Part model, mm, in its own coordinate system. Face numbers are marked on the shaded views. A direction names the side the tool comes from. Coordinates: 2 decimals unless noted, no trailing zeros. Write each loop counter-clockwise with the first axis right and the second up, starting at its lowest first coordinate (ties: lowest second). Pieces come first, ordered by that corner, then holes. Notation, with made-up numbers: (36, -13.5) - (42, -13.5) arc R18 ccw to (42, 10.5) - close; hole circle Ø6 at (5.25, 28.5). An arc over 180 degrees is marked (long way). Use one line per item in the form item = value. Start each with the question number.
from build123d import *

# Parameters (mm, degrees)
BOSS_EXTRUDE1_DEPTH = 15
CHAMFER1_SIZE       = 3
CHAMFER2_SIZE       = 3
SKETCH2_R           = 2.5
CUT_EXTRUDE1_DEPTH  = 37
SKETCH3_R           = 1.5
CUT_EXTRUDE2_DEPTH  = 6


with BuildPart() as part:
    # Sketch1 → Boss-Extrude1 (new body)
    with BuildSketch(Plane.XY):
        Polygon((8.117882489, 6.249295775), (12.117882489, 6.249295775), (12.117882489, -17.750704225), (-12.882117511, -17.750704225), (-12.882117511, 6.249295775), (-8.882117511, 6.249295775), (-8.882117511, -13.750704225), (8.117882489, -13.750704225), align=None)
    extrude(amount=BOSS_EXTRUDE1_DEPTH)

    # Chamfer1
    chamfer1_edges = [part.edges().sort_by_distance(p)[0] for p in [
        (-8.882117511, -13.750704225, 7.5),
    ]]
    chamfer(chamfer1_edges, length=CHAMFER1_SIZE)

    # Chamfer2
    chamfer2_edges = [part.edges().sort_by_distance(p)[0] for p in [
        (8.117882489, -13.750704225, 7.5),
    ]]
    chamfer(chamfer2_edges, length=CHAMFER2_SIZE)

    # Sketch2 → Cut-Extrude1 (cut)
    with BuildSketch(Plane.ZY.offset(12.882117511)):
        with Locations(Location((7.5, 1.249295775, 0), (0, 0, 90))):
            Circle(SKETCH2_R)
    extrude(amount=-CUT_EXTRUDE1_DEPTH, mode=Mode.SUBTRACT)

    # Sketch3 → Cut-Extrude2 (cut)
    with BuildSketch(Plane.XZ.offset(17.750704225)):
        with Locations(Location((-9.882117511, 12, 0), (0, 0, 270))):
            Circle(SKETCH3_R)
        with Locations(Location((-9.882117511, 3, 0), (0, 0, 90))):
            Circle(SKETCH3_R)
        with Locations(Location((9.117882489, 12, 0), (0, 0, 90))):
            Circle(SKETCH3_R)
        with Locations(Location((9.117882489, 3, 0), (0, 0, 270))):
            Circle(SKETCH3_R)
    extrude(amount=-CUT_EXTRUDE2_DEPTH, mode=Mode.SUBTRACT)


solid = part.part
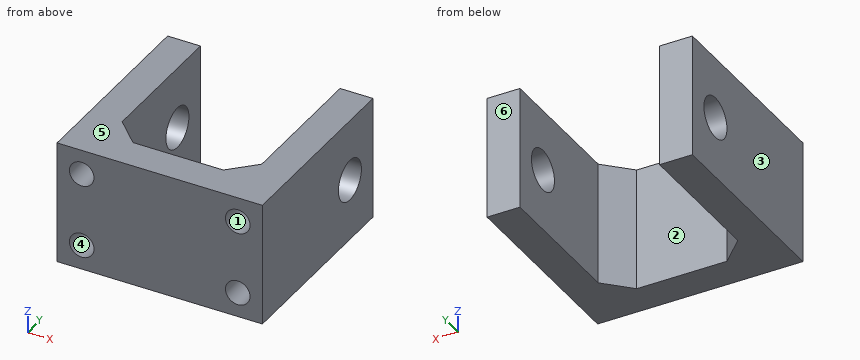
Q1. Pin check, flat tips, straight feed: P1, Ø2.5, axis at x = -10.5, z = 12, coming from the -Y side; P2, Ø0.9, axis at x = 9.5, z = 11.5, coming from the -Y side; P3, Ø9, axis at x = 2, z = 6.5, coming from the +Y side. Stop position of each tip, or through.
Q2. Slice it at B-B (y = 2). List the corners of the cut face in (x, z), plus the area to 3 significant figures.
Q3. Which spindle directions (+Z, -Z, +X, -X, +Y, -Y) get a long thin tool onto all of the face, cutting with end or side? Do the marked faces 1, 2 and 3. Say none if no direction does.
Q4. Slice it at D-D (x = 8.5). List the corners of the cut face in (y, z), plus the area to 3 significant figures.
Q5. Slice it at C-C (z = 3). List the corners of the cut face in (x, y), plus the area to 3 significant figures.
Q6. Slice it at A-A (z = 7.5). List the corners of the cut face in (x, y), plus the area to 3 significant figures.
Q7. Drill centre lines: probe 1 along X at (y, z) = (-14.2, 12); probe 2 along X at (y, z) = (-8, 8); probe 3 along X at (y, z) = (-13.2, 3). Where is each one in solid material? Low to high.
Q8. Mould opens along Z. For the marked faces 4, 5 and 6 say: released by +Z, released by -Z, zero draft, split by the parting line, or undercut.
Solution:
q1.P1 = -17.75
q1.P2 = -11.75
q1.P3 = -12.37
q2.outline = (-12.88, 0) - (-8.88, 0) - (-8.88, 5.12) - (-12.88, 5.12) - close; (-12.88, 9.88) - (-8.88, 9.88) - (-8.88, 15) - (-12.88, 15) - close; (8.12, 0) - (12.12, 0) - (12.12, 5.12) - (8.12, 5.12) - close; (8.12, 9.88) - (12.12, 9.88) - (12.12, 15) - (8.12, 15) - close
q2.area = 81.8 mm2
q3.face_1 = -Y
q3.face_2 = +Z, -Z, +Y
q3.face_3 = +Z, -Z, -X, +Y, -Y
q4.outline = (-17.75, 0) - (6.25, 0) - (6.25, 15) - (-17.75, 15) - (-17.75, 13.37) - (-11.75, 13.37) - (-11.75, 10.63) - (-17.75, 10.63) - (-17.75, 4.37) - (-11.75, 4.37) - (-11.75, 1.63) - (-17.75, 1.63) - close; hole circle Ø5 at (1.25, 7.5)
q4.area = 308 mm2
q5.outline = (-12.88, -17.75) - (-11.38, -17.75) - (-11.38, -11.75) - (-8.38, -11.75) - (-8.38, -17.75) - (7.62, -17.75) - (7.62, -11.75) - (10.62, -11.75) - (10.62, -17.75) - (12.12, -17.75) - (12.12, 6.25) - (8.12, 6.25) - (8.12, -10.75) - (5.12, -13.75) - (-5.88, -13.75) - (-8.88, -10.75) - (-8.88, 6.25) - (-12.88, 6.25) - close
q5.area = 233 mm2
q6.outline = (-12.88, -17.75) - (12.12, -17.75) - (12.12, -1.25) - (8.12, -1.25) - (8.12, -10.75) - (5.12, -13.75) - (-5.88, -13.75) - (-8.88, -10.75) - (-8.88, -1.25) - (-12.88, -1.25) - close; (-12.88, 3.75) - (-8.88, 3.75) - (-8.88, 6.25) - (-12.88, 6.25) - close; (8.12, 3.75) - (12.12, 3.75) - (12.12, 6.25) - (8.12, 6.25) - close
q6.area = 229 mm2
q7.probe_1 = -12.88 to -11.38, -8.38 to 7.62, 10.62 to 12.12
q7.probe_2 = -12.88 to -8.88, 8.12 to 12.12
q7.probe_3 = -12.88 to -11.38, -8.38 to -6.43, 5.67 to 7.62, 10.62 to 12.12
q8.face_4 = undercut
q8.face_5 = released by +Z
q8.face_6 = zero draft
